Could you check a few things on this drawing? It's one solid part, dimensions in mm from its lowest x, y, z. A direction names the side the tool comes from. Round coordinates to 2 decimals unless told otherwise and drop trailing zeros. Order: outer loops, then holes, each group sorted by start corner. A loop starts at its lowest first (then second) coordinate and runs counter-clockwise, first axis right, second up. Notation, with made-up numbers: M 67,-21 L 92,-21 A22 cw 92,7 Z; hole C 12,38.25 d3. An arc over 180 degrees is marked long. Answer as a JSON object with one key per item and string values. Group by question number.
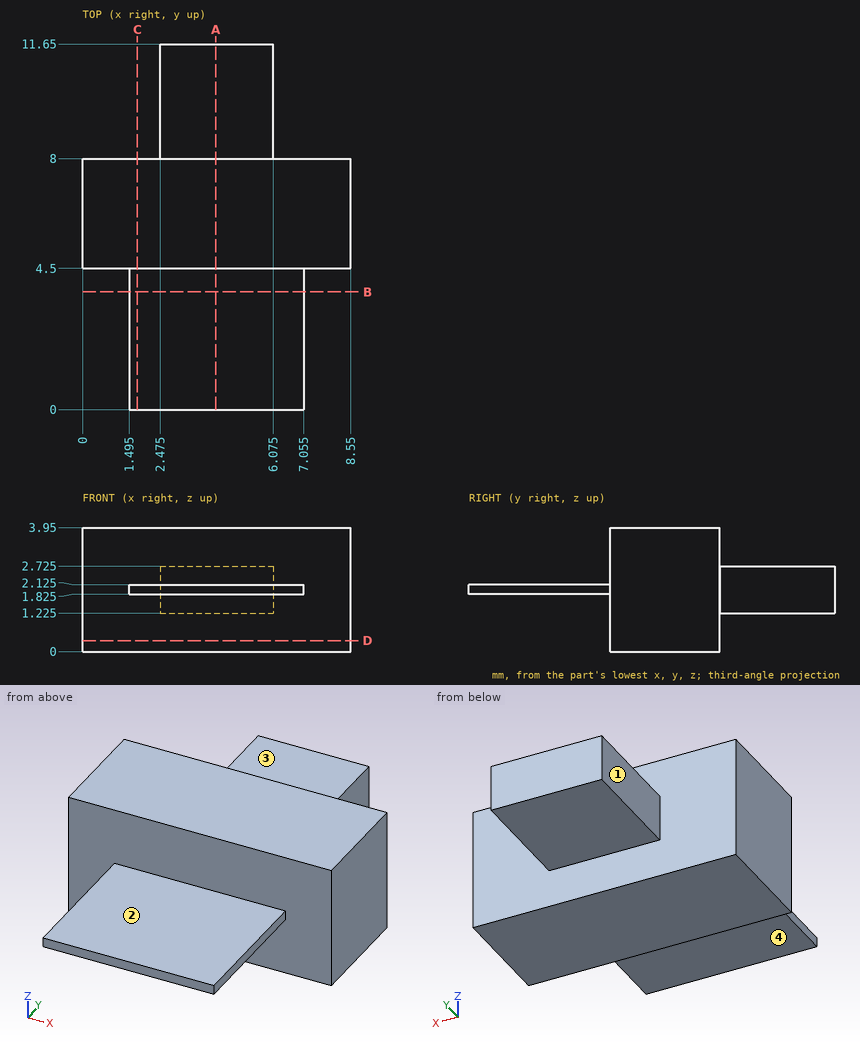
1) If we section it at A-A on x = 4.25: Write out the boundary of the cut face in (y, z) (3 decimals), plus the area to 4 significant figures.
2) If we section it at C-C on x = 1.75: Write out the boundary of the cut face in (y, z) (3 decimals).
3) Which directions (+Z, -Z, +X, -X, +Y, -Y) give clear straight access to the entire face, cutting with the end or side of a thin tool? Please do the marked faces 1, 2, 3 and 4.
4) For pin 1 (1.5 mm diameter, centred on y = 10, z = 1, fed in from +X) (3 decimals); pin 2 (1.8 mm diameter, centred on x = 5, y = 10, fed in from -Z) (3 decimals); pin 3 (2 mm diameter, centred on x = 3.5, y = 2, fed in from +Z) (3 decimals), each with a flat end and sliding along its axis, tell me the tip position at first contact or that it passes through.
5) If we section it at D-D on z = 0.35: Write out the boundary of the cut face in (x, y).
6) I need wall thicknesses on line 1 along Y through (x, z) = (2.25, 1.65); line 2 along Z through (x, y) = (4.5, 1) (3 decimals); line 3 along Y through (x, z) = (4.5, 1.7). Which ranges of each line are inside material? Lowest first, please.
7) If we section it at B-B on y = 3.75: Write out the boundary of the cut face in (x, z) (3 decimals), plus the area to 3 significant figures.
Findings:
{
 "1": {"outline": "M 0,1.825 L 4.5,1.825 L 4.5,0 L 8,0 L 8,1.225 L 11.65,1.225 L 11.65,2.725 L 8,2.725 L 8,3.95 L 4.5,3.95 L 4.5,2.125 L 0,2.125 Z", "area": "20.65 mm^2"},
 "2": {"outline": "M 0,1.825 L 4.5,1.825 L 4.5,0 L 8,0 L 8,3.95 L 4.5,3.95 L 4.5,2.125 L 0,2.125 Z"},
 "3": {"face 1": "+Z, -Z, -X, +Y", "face 2": "+Z, +X, -X, -Y", "face 3": "+Z, +X, -X, +Y", "face 4": "-Z, +X, -X, -Y"},
 "4": {"pin 1": "stops at x = 6.075", "pin 2": "stops at z = 1.225", "pin 3": "stops at z = 2.125"},
 "5": {"outline": "M 0,4.5 L 8.55,4.5 L 8.55,8 L 0,8 Z"},
 "6": {"line 1": "y = 4.5 to 8", "line 2": "z = 1.825 to 2.125", "line 3": "y = 4.5 to 11.65"},
 "7": {"outline": "M 1.495,1.825 L 7.055,1.825 L 7.055,2.125 L 1.495,2.125 Z", "area": "1.67 mm^2"}
}
